Autodesk Inventor part; units mm, degrees
ref_plane "YZ Plane" through (0, 0, 0) normal (1, 0, 0) x (0, 1, 0)
ref_plane "XZ Plane" through (0, 0, 0) normal (0, 1, 0) x (-1, 0, 0)
ref_plane "XY Plane" through (0, 0, 0) normal (0, 0, 1) x (1, 0, 0)
sketch "Sketch1" plane through (0, 0, 0) normal (0, 0, 1) x (1, 0, 0)
  line L0 (-11.658, 3.4387) -> (-11.658, -28.3113)
  line L1 (-11.658, 3.4387) -> (108.992, 3.4387)
  line L2 (108.992, 3.4387) -> (108.992, -28.3113)
  line L3 (108.992, -28.3113) -> (-11.658, -28.3113)
  point P0 (0, 0)
  dimension "d0" = 31.75
  dimension "d1" = 120.65
  dimension "d2" = 31.75
extrude "Extrusion1" add sketch "Sketch1" along normal blind 6.35
sketch "Sketch2" plane through (0, 0, 6.35) normal (0, 0, 1) x (1, 0, 0)
  line L0 (-11.658, 3.4387) -> (-11.658, -28.3113)
  line L1 (-11.658, -28.3113) -> (108.992, -28.3113)
  line L2 (108.992, -28.3113) -> (108.992, 3.4387)
  line L3 (-11.658, -28.3113) -> (-11.658, -21.9613)
  line L4 (-11.658, -21.9613) -> (108.992, -21.9613)
  line L5 (108.992, -28.3113) -> (-11.658, -28.3113)
  point P0 (0, 0)
  dimension "d5" = 6.35
extrude "Extrusion2" add sketch "Sketch2" along normal blind 25.4
sketch "Sketch3" plane through (-11.658, -21.9613, 6.35) normal (0, 1, 0) x (1, 0, 0)
  line L0 (0, 0) -> (120.65, 0)
  line L1 (120.65, -25.4) -> (0, -25.4)
  line L2 (120.65, 0) -> (120.65, -25.4)
  line L3 (0, -25.4) -> (12.7, -25.4)
  line L4 (12.7, -25.4) -> (12.7, 0)
  line L5 (12.7, 0) -> (19.05, 0)
  line L6 (19.05, 0) -> (19.05, -25.4)
  line L7 (19.05, -25.4) -> (12.7, -25.4)
  line L8 (19.05, -25.4) -> (63.5, -25.4)
  line L9 (63.5, -25.4) -> (63.5, 0)
  line L10 (63.5, 0) -> (69.85, 0)
  line L11 (69.85, 0) -> (69.85, -25.4)
  line L12 (69.85, -25.4) -> (63.5, -25.4)
  line L13 (69.85, -25.4) -> (114.3, -25.4)
  line L14 (114.3, -25.4) -> (114.3, 0)
  line L15 (120.65, 0) -> (114.3, 0)
  line L16 (120.65, 0) -> (120.65, -25.4)
  line L17 (114.3, -25.4) -> (120.65, -25.4)
  point P0 (11.658, 6.35)
  dimension "d8" = 12.7
  dimension "d9" = 6.35
  dimension "d10" = 25.4
  dimension "d11" = 44.45
  dimension "d12" = 6.35
  dimension "d13" = 25.4
  dimension "d14" = 44.45
extrude "Extrusion3" add sketch "Sketch3" along normal blind 25.4 contours L0 L6 L1 L4 | L0 L11 L1 L9 | L0 L2 L1 L14
sketch "Sketch4" plane through (7.392, -21.9613, 31.75) normal (1, 0, 0) x (0, 0, -1)
  line L0 (25.4, 0) -> (0, 0)
  line L1 (25.4, 25.4) -> (25.4, 0)
  line L2 (0, 25.4) -> (25.4, 25.4)
  line L3 (0, 0) -> (0, 25.4)
  point P0 (31.75, 21.9613)
sketch "Sketch5" plane through (108.992, -28.3113, 0) normal (1, 0, 0) x (0, 0, -1)
  line L0 (-31.75, 0) -> (-31.75, 31.75)
  line L1 (-31.75, 31.75) -> (-31.75, 19.05)
  line L2 (-31.75, 19.05) -> (-19.05, 19.05)
  circle A0 centre (-19.05, 19.05) radius 3.175
  point P0 (0, 28.3113)
  dimension "d17" = 12.7
  dimension "d18" = 12.7
  dimension "d19" = 6.35
extrude "Extrusion4" cut sketch "Sketch5" against normal blind 76.2
properties part number "corner"
For this review, take the finished solid that the model builds, in its own axes (mm). A direction names the side the tool comes from. Give positions to 0.01 mm unless a question says otherwise; leave off trailing zeros. Order: outer loops, then holes, each group sorted by start corner. A loop starts at its lowest first (then second) coordinate and runs counter-clockwise, first axis right, second up. Notation, with made-up numbers: (34, 2.5) -> (93, 2.5) arc R25 ccw to (93, 33.5) -> close; hole circle Ø10 at (68.5, 13). An arc over 180 degrees is marked (long way). Write item = value, one per line.
1) We need section D-D, the plane z = 8.5. Give the boundary of the cut face in (x, y).
Findings:
outline = (-11.66, -28.31) -> (108.99, -28.31) -> (108.99, 3.44) -> (102.64, 3.44) -> (102.64, -21.96) -> (58.19, -21.96) -> (58.19, 3.44) -> (51.84, 3.44) -> (51.84, -21.96) -> (7.39, -21.96) -> (7.39, 3.44) -> (1.04, 3.44) -> (1.04, -21.96) -> (-11.66, -21.96) -> close
2) For faces 5 (the face through (105.86, -8.31, 16.02)), 6 (the face through (7.392, -9, 19)), 7 (the face through (-5, -21.961, 19)), list the 3-axis set-ups (+Z, -Z, +X, -X, +Y, -Y) from which the entire face can be reached by the end or side of a thin tool; tool diameter is ignored.
Findings:
face_5 = +X
face_6 = +Z, +Y
face_7 = +Z, -X, +Y
3) We need section A-A, the plane z = 19.05. Give the boundary of the cut face in (x, y), and give its area (3 significant figures).
Findings:
outline = (-11.66, -28.31) -> (108.99, -28.31) -> (108.99, -12.44) -> (102.64, -12.44) -> (102.64, -21.96) -> (58.19, -21.96) -> (58.19, -12.44) -> (51.84, -12.44) -> (51.84, -21.96) -> (7.39, -21.96) -> (7.39, 3.44) -> (1.04, 3.44) -> (1.04, -21.96) -> (-11.66, -21.96) -> close; (51.84, -6.09) -> (58.19, -6.09) -> (58.19, 3.44) -> (51.84, 3.44) -> close; (102.64, -6.09) -> (108.99, -6.09) -> (108.99, 3.44) -> (102.64, 3.44) -> close
area = 1,170 mm^2
4) Draft analysis for pull direction X (two halves, no side actions). For faces 1 (the face through (108.992, -12, 16)), 2 (the face through (29, -21.961, 19)), 3 (the face through (-11.658, -23, 9)), 4 (the face through (55.06, -8.31, 16.02)), state which applies: pulls with the +X half, pulls with the -X half, needs draft (parallel to the pull), parting line crosses it, or undercut.
Findings:
face_1 = pulls with the +X half
face_2 = undercut
face_3 = pulls with the -X half
face_4 = needs draft
5) We need section B-B, the plane y = -20.5. Give the boundary of the cut face in (x, z).
Findings:
outline = (-11.66, 0) -> (108.99, 0) -> (108.99, 31.75) -> (102.64, 31.75) -> (102.64, 6.35) -> (58.19, 6.35) -> (58.19, 31.75) -> (51.84, 31.75) -> (51.84, 6.35) -> (7.39, 6.35) -> (7.39, 31.75) -> (1.04, 31.75) -> (1.04, 6.35) -> (-11.66, 6.35) -> close
6) To check wall thickness, follow L1, parallel to X at y = 0.5, z = 15; L2, parallel to Y at x = 39, z = 7.5; L3, parallel to Z at x = 97, y = -21.5. State the ranges of each line that lie inside material, in increasing order. Write a range as from..to.
Findings:
L1 = 1.04..7.39, 51.84..58.19, 102.64..108.99
L2 = -28.31..-21.96
L3 = 0..6.35
7) We need section C-C, the plane y = -11. Give the boundary of the cut face in (x, z), and give its area (3 significant figures).
Findings:
outline = (-11.66, 0) -> (108.99, 0) -> (108.99, 16.39) -> (102.64, 16.39) -> (102.64, 6.35) -> (58.19, 6.35) -> (58.19, 16.39) -> (51.84, 16.39) -> (51.84, 6.35) -> (7.39, 6.35) -> (7.39, 31.75) -> (1.04, 31.75) -> (1.04, 6.35) -> (-11.66, 6.35) -> close; (51.84, 21.71) -> (58.19, 21.71) -> (58.19, 31.75) -> (51.84, 31.75) -> close; (102.64, 21.71) -> (108.99, 21.71) -> (108.99, 31.75) -> (102.64, 31.75) -> close
area = 1,180 mm^2
8) Insertion check: pin 1 (10 mm diameter, centred on y = -9.26, z = 19.05, fed in from -X); pin 2 (14 mm diameter, centred on x = -8.5, z = 21.5, fed in from +Y); pin 3 (12.5 mm diameter, centred on x = 22.5, y = -9.5, fed in from +Z). Each pin has a flat end and moves straight along its axis. Give the tip position at first contact, or say it passes through.
Findings:
pin_1 = 1.04
pin_2 = -21.96
pin_3 = 6.35
